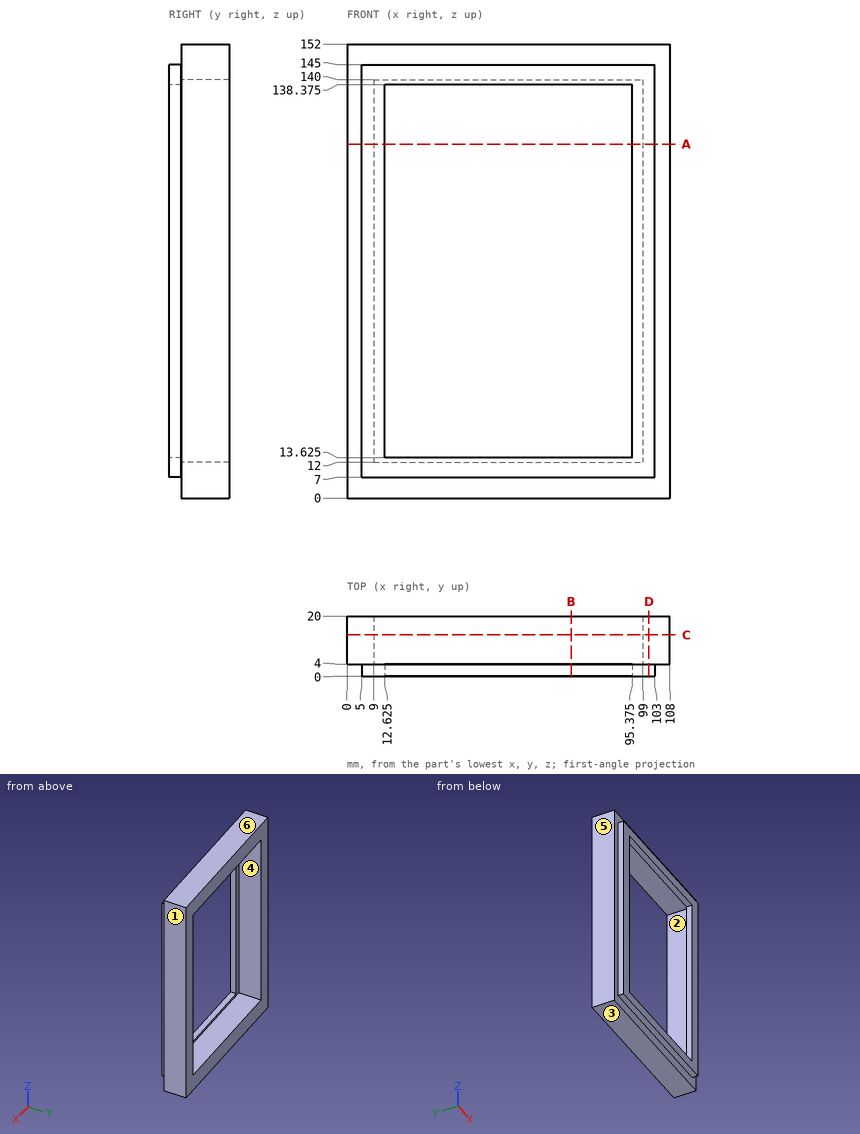
Here's the drawing with two shaded views (mm, measured from the low corner). I have some questions. A direction names the side the tool comes from. Round coordinates to 2 decimals unless told otherwise and drop trailing zeros. Loops run counter-clockwise (first coordinate to the right, second up) from the corner with the lowest first, then second, coordinate; pieces in that order, holes last.
Item 1: If we mould it in two halves opening along Z, with no side actions, what happens to the marked faces 3, 4, 5 and 6? For each: +Z half, -Z half, draft (parallel to the pull), parting line (faces both ways), or undercut.
Item 2: Please list where these lines run through material, in increasing order: L1, parallel to Z at x = 17, y = 12.5; L2, parallel to Z at x = 67, y = 3.5 (3 decimals); L3, parallel to X at y = 1.5, z = 56 (3 decimals).
Item 3: Suppose I cut it at C-C, the plane y = 13.75. Write out the boundary of the cut face in (x, z).
Item 4: Which directions (+Z, -Z, +X, -X, +Y, -Y) give clear straight access to the entire face, cutting with the end or side of a thin tool? Please do the marked faces 1 and 2.
Item 5: Suppose I cut it at D-D, the plane x = 101. Write out the boundary of the cut face in (y, z), then the cut area to 3 significant figures.
Item 6: Will these pins go through, and if not, where does the flat tip stop? pin 1 Ø1.5 at (y, z) = (3, 70) entering from +X; pin 2 Ø2 at (x, y) = (71, 1) entering from -Z; pin 3 Ø4.5 at (x, y) = (51.5, 1.5) entering from +Z.
Item 7: Suppose I cut it at B-B, the plane x = 75. Write out the boundary of the cut face in (y, z) (3 decimals).
Item 8: Suppose I cut it at A-A, the plane z = 118.5. Write out the boundary of the cut face in (x, y) (3 decimals), then the cut area to 3 significant figures.
Reported:
1. face 3: -Z half
1. face 4: undercut
1. face 5: draft
1. face 6: +Z half
2. L1: z = 0 to 12, 140 to 152
2. L2: z = 7 to 13.625, 138.375 to 145
2. L3: x = 5 to 12.625, 95.375 to 103
3. outline: (0, 0) - (108, 0) - (108, 152) - (0, 152) - close; hole (9, 12) - (99, 12) - (99, 140) - (9, 140) - close
4. face 1: +Z, -Z, +X, +Y, -Y
4. face 2: +Y
5. outline: (0, 7) - (4, 7) - (4, 0) - (20, 0) - (20, 152) - (4, 152) - (4, 145) - (0, 145) - close
5. area: 2,980 mm2
6. pin 1: stops at x = 103
6. pin 2: stops at z = 7
6. pin 3: stops at z = 145
7. outline: (0, 7) - (4, 7) - (4, 0) - (20, 0) - (20, 12) - (4, 12) - (4, 13.625) - (0, 13.625) - close; (0, 138.375) - (4, 138.375) - (4, 140) - (20, 140) - (20, 152) - (4, 152) - (4, 145) - (0, 145) - close
8. outline: (0, 4) - (5, 4) - (5, 0) - (12.625, 0) - (12.625, 4) - (9, 4) - (9, 20) - (0, 20) - close; (95.375, 0) - (103, 0) - (103, 4) - (108, 4) - (108, 20) - (99, 20) - (99, 4) - (95.375, 4) - close
8. area: 349 mm2
